```python
from build123d import *

# Parameters (mm, degrees)
RESSALTO_EXTRUS_O1_DEPTH = 6.35
ESBO_O2_R                = 10.975
ESBO_O2_R_2              = 2.5
CORTE_EXTRUS_O1_DEPTH    = 28.62489819
CORTE_EXTRUS_O2_DEPTH    = 28.62489819
ESBO_O4_W                = 5
ESBO_O4_H                = 0.2
CORTE_EXTRUS_O3_DEPTH    = 28.62489819


with BuildPart() as part:
    # Esboço1 → Ressalto-extrusão1 (new body)
    with BuildSketch(Plane.XY):
        with BuildLine():
            Line((-20.578767123, 4.424572712), (-6.287671233, 11.946346323))
            ThreePointArc((-6.287671233, 11.946346323), (0, 13.5), (6.287671233, 11.946346323))
            Line((6.287671233, 11.946346323), (20.578767123, 4.424572712))
            ThreePointArc((20.578767123, 4.424572712), (23.25, 0), (20.578767123, -4.424572712))
            Line((20.578767123, -4.424572712), (6.287671233, -11.946346323))
            ThreePointArc((6.287671233, -11.946346323), (0, -13.5), (-6.287671233, -11.946346323))
            Line((-6.287671233, -11.946346323), (-20.578767123, -4.424572712))
            ThreePointArc((-20.578767123, -4.424572712), (-23.25, 0), (-20.578767123, 4.424572712))
        make_face()
    extrude(amount=RESSALTO_EXTRUS_O1_DEPTH)

    # Esboço2 → Corte-extrusão1 (cut, through all)
    with BuildSketch(Plane.XY.offset(6.35)):
        Circle(ESBO_O2_R)
        with Locations((-18.25, 0)):
            Circle(ESBO_O2_R_2)
        with Locations((18.25, 0)):
            Circle(ESBO_O2_R_2)
    extrude(amount=-CORTE_EXTRUS_O1_DEPTH, mode=Mode.SUBTRACT)

    # Esboço3 → Corte-extrusão2 (cut, through all)
    with BuildSketch(Plane.XY.offset(6.35)):
        with BuildLine():
            Line((0.1, -10.97454441), (0.1, -13.499629625))
            ThreePointArc((0.1, -13.499629625), (0, -13.5), (-0.1, -13.499629625))
            Line((-0.1, -13.499629625), (-0.1, -10.97454441))
            ThreePointArc((-0.1, -10.97454441), (0, -10.975), (0.1, -10.97454441))
        make_face()
    extrude(amount=-CORTE_EXTRUS_O2_DEPTH, mode=Mode.SUBTRACT)

    # Esboço4 → Corte-extrusão3 (cut, through all)
    with BuildSketch(Plane.XY.offset(6.35)):
        with Locations((-20.75, 0)):
            Rectangle(ESBO_O4_W, ESBO_O4_H)
    corte_extrus_o3 = extrude(amount=-CORTE_EXTRUS_O3_DEPTH, mode=Mode.SUBTRACT)

    # Espelhar1: Corte-extrusão3 across plane
    add(corte_extrus_o3.mirror(Plane(origin=(0, 0, 0), x_dir=(0, 0, 1), z_dir=(1, 0, 0))), mode=Mode.SUBTRACT)


solid = part.part
```
Input: part model. Units: mm. Frame: model coordinates. A direction names the side the tool comes from. Coordinates: 2 decimals unless noted, no trailing zeros. Loops run counter-clockwise (first coordinate to the right, second up) from the corner with the lowest first, then second, coordinate; pieces in that order, holes last. Notation, with made-up numbers: M 15,24.5 L 55,24.5 A32 ccw 55,61.5 Z; hole C 21,39 d7. An arc over 180 degrees is marked long. Use a Markdown table: item, result. Add a question column.
1) Section A-A, the plane x = 10. Return the cut outline in (y, z), plus the area to 3 significant figures.
2) Set-up query: faces 1 (the flat face through (-0.1, -12, 3)), 2 (the flat face through (22, 0.1, 3)), 3 (the flat face through (13.533, -8.133, 3.131)). Return all of +Z, -Z, +X, -X, +Y, -Y with unobstructed straight access to the full face (end or side cutting, diameter ignored); none if empty.
3) Draft query along Y for faces 4 (the flat face through (-22, 0.1, 3)), 5 (the cylindrical face through (-22.485, -2.659, 3.131)), 6 (the flat face through (-22, -0.1, 3)), 7 (the cylindrical face through (22.485, 2.659, 3.131)). Return one class per face: +Y half, -Y half, draft (parallel to the pull), parting line (faces both ways), or undercut.
4) Line query: L1, parallel to X at y = 0, z = 3 (3 decimals); L2, parallel to Y at x = 19, z = 1.5; L3, parallel to X at y = 3.75, z = 4.25. Output: solid intervals per line, ascending. Write a range as from..to.
5) Section C-C, the plane z = 4. Return the cut outline in (x, y) (3 decimals), plus the area to 3 significant figures.
6) Pin query (flat end, axial travel): P1, Ø2, axis at x = -17.5, z = 4.5, coming from the -Y side; P2, Ø0.8, axis at y = -11.5, z = 3, coming from the +X side; P3, Ø1.3, axis at x = -21.5, z = 3.5, coming from the -Y side. Return the tip coordinate at first contact, or that it passes through.
7) Section B-B, the plane y = -9.5. Return the cut outline in (x, z).
Answer below:
| question | item | result |
|---|---|---|
| 1 | outline | M -9.99,0 L -4.52,0 L -4.52,6.35 L -9.99,6.35 Z; M 4.52,0 L 9.99,0 L 9.99,6.35 L 4.52,6.35 Z |
| 1 | area | 69.5 mm2 |
| 2 | face 1 | +Z, -Z, -Y |
| 2 | face 2 | +Z, -Z, +X |
| 2 | face 3 | +Z, -Z, +X, -Y |
| 3 | face 4 | undercut |
| 3 | face 5 | -Y half |
| 3 | face 6 | undercut |
| 3 | face 7 | +Y half |
| 4 | L1 | -15.75..-10.975, 10.975..15.75 |
| 4 | L2 | -5.26..-2.38, 2.38..5.26 |
| 4 | L3 | -21.56..-10.31, 10.31..21.56 |
| 5 | outline | M -23.249,-0.1 A5 ccw -20.579,-4.425 L -6.288,-11.946 A13.5 ccw -0.1,-13.5 L -0.1,-10.975 A10.975 cw long 0.1,-10.975 L 0.1,-13.5 A13.5 ccw 6.288,-11.946 L 20.579,-4.425 A5 ccw 23.249,-0.1 L 20.748,-0.1 A2.5 cw long 20.748,0.1 L 23.249,0.1 A5 ccw 20.579,4.425 L 6.288,11.946 A13.5 ccw -6.288,11.946 L -20.579,4.425 A5 ccw -23.249,0.1 L -20.748,0.1 A2.5 cw long -20.748,-0.1 Z |
| 5 | area | 409 mm2 |
| 6 | P1 | y = -6.57 |
| 6 | P2 | x = 7.9 |
| 6 | P3 | y = -4.27 |
| 7 | outline | M -10.94,0 L -5.5,0 L -5.5,6.35 L -10.94,6.35 Z; M 5.5,0 L 10.94,0 L 10.94,6.35 L 5.5,6.35 Z |
